Could you check a few things on this drawing? It's one solid part, dimensions in mm from its lowest x, y, z. Give positions to 0.01 mm unless a question says otherwise; leave off trailing zeros. Order: outer loops, then holes, each group sorted by start corner. A loop starts at its lowest first (then second) coordinate and runs counter-clockwise, first axis right, second up. Notation, with made-up numbers: M 81.5,74 L 119.5,74 A35 cw 119.5,113 Z; hole C -34,-12 d2. An arc over 180 degrees is marked long. Use one line per item in the form item = value. Start each with the question number.
1. I need wall thicknesses on L1, parallel to Z at x = 196.5, y = 170 (1 decimal); L2, parallel to Y at x = 359.5, z = 254; L3, parallel to Y at x = 212, z = 207.5 (1 decimal). Which ranges of each line are inside material? Lowest first, please.
2. I want a section at A-A, the plane x = 493.5. List the corners of the cut face in (y, z) for me (1 decimal).
3. I want a section at B-B, the plane y = 250. List the corners of the cut face in (x, z) for me (1 decimal).
4. We'd pull the mould along Y, two halves only. Please class the marked faces 1, 2 and 3: +Y half, -Y half, draft (parallel to the pull), parting line (faces both ways), or undercut.
5. I want a section at D-D, the plane y = 66. List the corners of the cut face in (x, z) for me.
6. I want a section at C-C, the plane z = 291. List the corners of the cut face in (x, y) for me, and give its area (3 significant figures).
7. Will these pins go through, and if not, where does the flat tip stop? P1, Ø3, axis at x = 82, y = 84.5, coming from the +Z side; P2, Ø1, axis at x = 425, y = 133, coming from the -Z side; P3, Ø10, axis at x = 338, z = 179.5, coming from the +Y side; P4, Ø12, axis at x = 239, z = 242.5, coming from the +Y side (1 decimal).
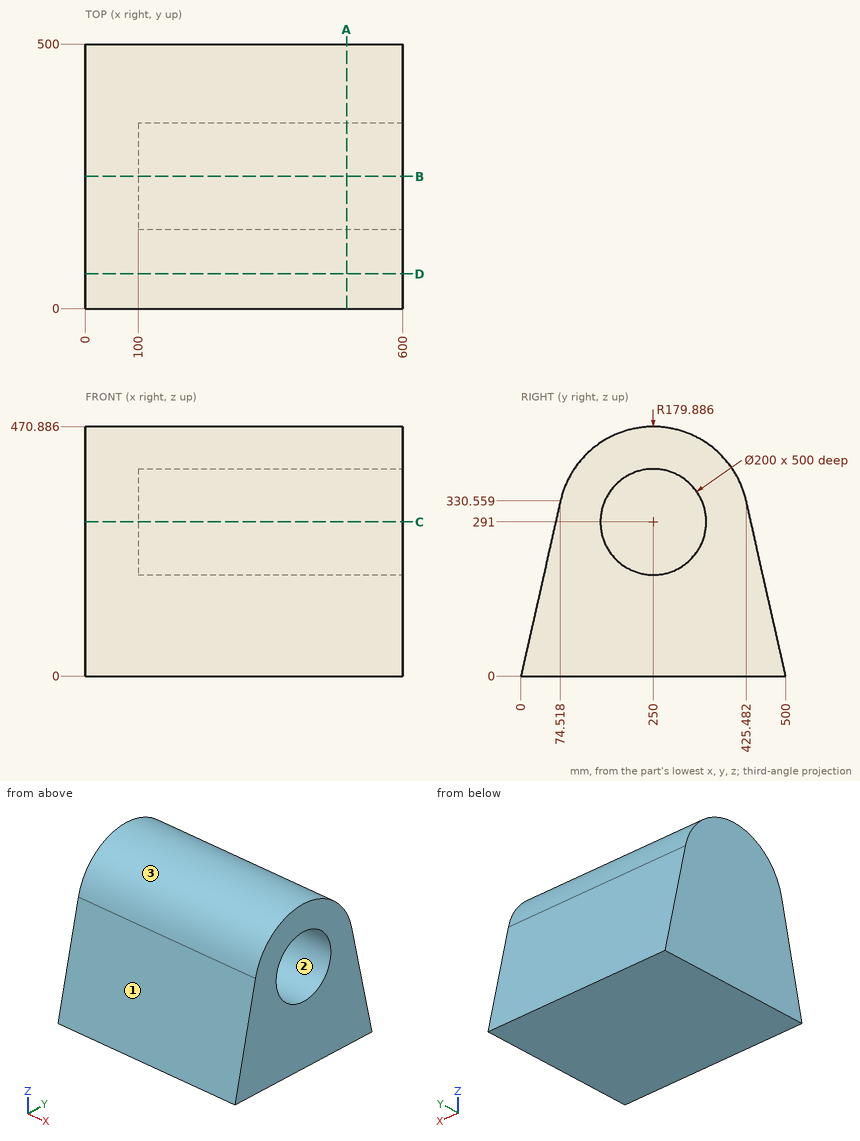
Check result:
q1.L1 = 0 to 231, 351 to 452.1
q1.L2 = 57.26 to 157.1, 342.9 to 442.74
q1.L3 = 46.8 to 195, 305 to 453.2
q2.outline = M 0,0 L 500,0 L 425.5,330.6 A179.9 ccw 74.5,330.6 Z; hole C 250,291 d200
q3.outline = M 0,0 L 600,0 L 600,191 L 100,191 L 100,391 L 600,391 L 600,470.9 L 0,470.9 Z
q4.face_1 = -Y half
q4.face_2 = undercut
q4.face_3 = parting line
q5.outline = M 0,0 L 600,0 L 600,292.77 L 0,292.77 Z
q6.outline = M 0,65.6 L 600,65.6 L 600,150 L 100,150 L 100,350 L 600,350 L 600,434.4 L 0,434.4 Z
q6.area = 121,000 mm2
q7.P1 = 364.91
q7.P2 = 0
q7.P3 = 460.66
q7.P4 = 446.7
